The listing builds one solid part. Answer for the finished solid, in the listing's coordinates (mm). Face numbers are marked on the shaded views. Give positions to 0.01 mm unless a question says otherwise; leave off trailing zeros. Order: outer loops, then holes, each group sorted by start corner. A loop starts at its lowest first (then second) coordinate and runs counter-clockwise, first axis right, second up.
```python
from build123d import *

# Parameters (mm, degrees)
CROQUIS1_R              = 0.999999899
CROQUIS1_R_2            = 0.999998866
CROQUIS1_R_3            = 1.000000014
CROQUIS1_R_4            = 0.999999985
SALIENTE_EXTRUIR1_DEPTH = 3
SALIENTE_EXTRUIR2_REACH = 38.281
CROQUIS3_W              = 35.45
CROQUIS3_H              = 2.45
SALIENTE_EXTRUIR3_DEPTH = 3
CROQUIS4_R              = 0.999999985
CROQUIS4_R_2            = 1.000000014
CORTAR_EXTRUIR1_DEPTH   = 17
CORTAR_EXTRUIR2_DEPTH   = 31
REDONDEO1_R             = 3


with BuildPart() as part:
    # Croquis1 → Saliente-Extruir1 (new body)
    with BuildSketch(Plane(origin=(0, 0, 0), x_dir=(1, 0, 0), z_dir=(0, 1, 0))):
        Polygon((25.246177886, -7.147133033), (25.246177886, 7.827867349), (15.296177123, 5.340367158), (15.296177123, 12.840367158), (-26.15382364, 12.790366967), (-26.15382364, -12.109632651), (15.296177123, -12.159632842), (15.296177123, -4.659632842), align=None)
        with Locations(Location((9.246177066, 6.34036702, 0), (0, 0, 270))):
            Circle(CROQUIS1_R, mode=Mode.SUBTRACT)
        with Locations(Location((9.246182607, -5.65963638, 0), (0, 0, 270))):
            Circle(CROQUIS1_R_2, mode=Mode.SUBTRACT)
        with Locations(Location((-20.153822905, -5.659632902, 0), (0, 0, 270))):
            Circle(CROQUIS1_R_3, mode=Mode.SUBTRACT)
        with Locations(Location((-20.15382331, 6.340367521, 0), (0, 0, 270))):
            Circle(CROQUIS1_R_4, mode=Mode.SUBTRACT)
    extrude(amount=SALIENTE_EXTRUIR1_DEPTH)

    # Saliente-Extruir2: up to this plane
    saliente_extruir2_end = Plane(origin=(15.296177123, 3, -12.840367158), z_dir=(0.0012062763193973866, 0, 0.999999272448456))
    # Croquis2 → Saliente-Extruir2 (add, up to the surface)
    with BuildSketch(Plane(origin=(-0.014645609, 0, 12.141163746), x_dir=(0.999999272448456, 0, 0.0012062763194219445), z_dir=(-0.0012062763194219447, 0, 0.999999272448456)), mode=Mode.PRIVATE) as saliente_extruir2_sk1:
        with BuildLine():
            Line((-25.335349472, 3), (-14.943044626, 3))
            ThreePointArc((-14.943044626, 3), (-20.139197049, 6), (-25.335349472, 3))
        make_face()
    saliente_extruir2_tool1 = split(extrude(saliente_extruir2_sk1.sketch, amount=-SALIENTE_EXTRUIR2_REACH, mode=Mode.PRIVATE), bisect_by=saliente_extruir2_end, keep=Keep.BOTH, mode=Mode.PRIVATE)
    add(saliente_extruir2_tool1.solids().sort_by_distance((-20.153828, 4.230121, 12.11687))[0])

    # Croquis3 → Saliente-Extruir3 (add)
    with BuildSketch(Plane(origin=(0, 3, 0), x_dir=(1, 0, 0), z_dir=(0, 1, 0))):
        with Locations((-2.428822877, -10.934632842)):
            Rectangle(CROQUIS3_W, CROQUIS3_H)
        with Locations((-2.428822877, 11.615367158)):
            Rectangle(CROQUIS3_W, CROQUIS3_H)
    extrude(amount=SALIENTE_EXTRUIR3_DEPTH)

    # Croquis4 → Cortar-Extruir1 (cut)
    with BuildSketch(Plane.XZ):
        with Locations(Location((-20.15382331, -6.340367521, 0), (0, 0, 270))):
            Circle(CROQUIS4_R)
        with Locations(Location((-20.153822905, 5.659632902, 0), (0, 0, 270))):
            Circle(CROQUIS4_R_2)
    extrude(amount=-CORTAR_EXTRUIR1_DEPTH, mode=Mode.SUBTRACT)

    # Croquis5 → Cortar-Extruir2 (cut)
    with BuildSketch(Plane(origin=(-0.014645609, 0, 12.141163746), x_dir=(0.999999272448456, 0, 0.0012062763194219445), z_dir=(-0.0012062763194219447, 0, 0.999999272448456))):
        with BuildLine():
            Line((-20.139197049, 6), (-20.139197049, 8.549534658))
            ThreePointArc((-20.139197049, 8.549534658), (-26.184630981, 6.045433933), (-28.688731707, 0))
            Line((-28.688731707, 0), (-26.139197049, 0))
            ThreePointArc((-26.139197049, 0), (-24.381837736, 4.242640687), (-20.139197049, 6))
        make_face()
    extrude(amount=-CORTAR_EXTRUIR2_DEPTH, mode=Mode.SUBTRACT)

    # Redondeo1
    redondeo1_edges = [part.edges().sort_by_distance(p)[0] for p in [
        (-5.428823259, 0, 12.134632747),
        (-5.413805086, 0, -12.815385179),
    ]]
    fillet(redondeo1_edges, radius=REDONDEO1_R - 0.0001)  # a hair under: the kernel refuses the full size


solid = part.part
```
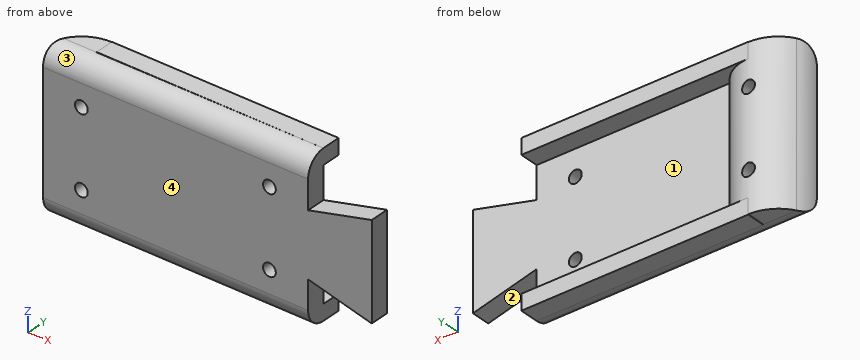
1) Find section C-C (x = 21). Write down the section's boundary in (y, z), then the cut area to 3 significant figures.
Geometry says:
outline: (0, -6.77) - (3, -6.77) - (3, 6.09) - (0, 6.09) - close
area: 38.6 mm2
2) Find section B-B (y = 0.75). Write down the section's boundary in (x, z).
Geometry says:
outline: (-26.11, 11.09) - (-26.08, -11.77) - (15.3, -11.82) - (15.3, -5.34) - (25.25, -7.83) - (25.25, 7.15) - (15.3, 4.66) - (15.3, 11.14) - close; hole circle Ø2 at (-20.15, -6.34); hole circle Ø2 at (-20.15, 5.66); hole circle Ø2 at (9.25, -6.34); hole circle Ø2 at (9.25, 5.66)
3) For a pull along Z with two mould halves and no side action, classify the marked faces 1, 2, 3 and 4 as +Z half, -Z half, draft (parallel to the pull), parting line (faces both ways), or undercut.
Geometry says:
face 1: undercut
face 2: -Z half
face 3: +Z half
face 4: draft
4) Given P1, Ø2.5, axis at x = 9.25, z = 5.66, coming from the +Y side; P2, Ø1, axis at y = 2, z = 8, coming from the +X side; P3, Ø1, axis at y = 5, z = -3, coming from the +X side, each flat-ended and moving along its own axis, determine where each tip first touches the part or whether it passes through.
Geometry says:
P1: stops at y = 3
P2: stops at x = 15.3
P3: stops at x = -16.17
5) Find section A-A (y = 3.5). Write down the section's boundary in (x, z), then the cut area to 3 significant figures.
Geometry says:
outline: (-25.03, 12.11) - (-25, -12.79) - (-20.15, -12.8) - (-20.15, -12.84) - (15.3, -12.84) - (15.3, -10.39) - (-15.25, -10.39) - (-15.28, 9.71) - (15.3, 9.71) - (15.3, 12.16) - (-20.15, 12.16) - (-20.15, 12.12) - close; hole circle Ø2 at (-20.15, -6.34); hole circle Ø2 at (-20.15, 5.66)
area: 387 mm2
